The model under review builds one solid part; all positions refer to its coordinate system, in mm. A direction names the side the tool comes from. Give positions to 0.01 mm unless a question says otherwise; leave off trailing zeros. Loops run counter-clockwise (first coordinate to the right, second up) from the corner with the lowest first, then second, coordinate; pieces in that order, holes last. Notation, with made-up numbers: (44, -35.75) - (57, -35.75) arc R24 cw to (57, 2.25) - close; hole circle Ø11 at (-19.5, 50.5). An arc over 180 degrees is marked (long way). Answer as a JSON object with one key per item and string values.
from build123d import *

# Parameters (mm, degrees)
ESQUISSE1_R        = 1.5
BOSS_EXTRU_1_DEPTH = 5


with BuildPart() as part:
    # Esquisse1 → Boss.-Extru.1 (new body)
    with BuildSketch(Plane.XY):
        with BuildLine():
            Line((18.252383146, -3.580169779), (18.252383146, 3.419830221))
            ThreePointArc((18.252383146, 3.419830221), (17.08081027, 6.248257345), (14.252383146, 7.419830221))
            Line((14.252383146, 7.419830221), (-12.747616854, 7.419830221))
            ThreePointArc((-12.747616854, 7.419830221), (-15.576043979, 6.248257345), (-16.747616854, 3.419830221))
            Line((-16.747616854, 3.419830221), (-16.747616854, -3.580169779))
            ThreePointArc((-16.747616854, -3.580169779), (-16.161830417, -4.994383342), (-14.747616854, -5.580169779))
            Line((-14.747616854, -5.580169779), (16.312383146, -5.580169779))
            ThreePointArc((16.312383146, -5.580169779), (17.687966708, -4.973585835), (18.252383146, -3.580169779))
        make_face()
        with Locations((13.582383146, -1.580169779)):
            Circle(ESQUISSE1_R, mode=Mode.SUBTRACT)
        with Locations((-12.017616854, -1.580169779)):
            Circle(ESQUISSE1_R, mode=Mode.SUBTRACT)
        with BuildLine():
            Line((-5.417616854, 1.919830221), (6.982383146, 1.919830221))
            ThreePointArc((6.982383146, 1.919830221), (8.482383146, 3.419830221), (6.982383146, 4.919830221))
            Line((6.982383146, 4.919830221), (-5.417616854, 4.919830221))
            ThreePointArc((-5.417616854, 4.919830221), (-6.917616854, 3.419830221), (-5.417616854, 1.919830221))
        make_face(mode=Mode.SUBTRACT)
    extrude(amount=BOSS_EXTRU_1_DEPTH)


solid = part.part
Q1. Consider section C-C, the plane x = -12. State the section outline as (y, z) points.
Results:
{"outline": "(-5.58, 0) - (-3.08, 0) - (-3.08, 5) - (-5.58, 5) - close; (-0.08, 0) - (7.42, 0) - (7.42, 5) - (-0.08, 5) - close"}
Q2. To check wall thickness, follow probe 1 along Y at (x, z) = (-5, 4.2); probe 2 along X at (y, z) = (-0.5, 2.75); probe 3 along X at (y, z) = (4.25, 0.3). State the ranges of each line that lie inside material, in increasing order. Write a range as [from, to].
Results:
{"probe 1": "y = [-5.58, 1.92], [4.92, 7.42]", "probe 2": "x = [-16.75, -13.06], [-10.98, 12.54], [14.62, 18.25]", "probe 3": "x = [-16.66, -6.67], [8.23, 18.17]"}
Q3. Consider section D-D, the plane y = 5.5. State the section outline as (x, z) points, plus the area to 3 significant figures.
Results:
{"outline": "(-16.16, 0) - (17.67, 0) - (17.67, 5) - (-16.16, 5) - close", "area": "169 mm^2"}
Q4. Consider section B-B, the plane z = 1.7. State the section outline as (x, y) points.
Results:
{"outline": "(-16.75, -3.58) arc R2 ccw to (-14.75, -5.58) - (16.31, -5.58) arc R2 ccw to (18.25, -3.58) - (18.25, 3.42) arc R4 ccw to (14.25, 7.42) - (-12.75, 7.42) arc R4 ccw to (-16.75, 3.42) - close; hole circle Ø3 at (-12.02, -1.58); hole (-5.42, 1.92) - (6.98, 1.92) arc R1.5 ccw to (6.98, 4.92) - (-5.42, 4.92) arc R1.5 ccw to start; hole circle Ø3 at (13.58, -1.58)"}
Q5. The part is to be moulded in two halves that separate along X. For faces 1 (the face through (-15.545, 6.279, 2.465)), 2 (the face through (1, 1, 5)), 3 (the face through (17.67, -4.99, 2.46)), 4 (the face through (12.084, -1.514, 2.465)), say which applies: +X half, -X half, draft (parallel to the pull), parting line (faces both ways), or undercut.
Results:
{"face 1": "-X half", "face 2": "draft", "face 3": "+X half", "face 4": "undercut"}
Q6. For faces 5 (the face through (1, -5.58, 2)), 6 (the face through (8.482, 3.387, 2.465)), list the 3-axis set-ups (+Z, -Z, +X, -X, +Y, -Y) from which the entire face can be reached by the end or side of a thin tool; tool diameter is ignored.
Results:
{"face 5": "+Z, -Z, +X, -X, -Y", "face 6": "+Z, -Z"}
Q7. Clearance check with a flat-ended pin moving along its axis: pin 1 Ø2.5 at (x, y) = (-12.02, -1.58) entering from +Z. State where the tip first meets the part, or that it passes through.
Results:
{"pin 1": "passes through"}
Q8. Consider section A-A, the plane x = 1. State the section outline as (y, z) points, plus the area to 3 significant figures.
Results:
{"outline": "(-5.58, 0) - (1.92, 0) - (1.92, 5) - (-5.58, 5) - close; (4.92, 0) - (7.42, 0) - (7.42, 5) - (4.92, 5) - close", "area": "50.0 mm^2"}
